Read the model definition and answer for the solid it produces. Units are mm, in the model's axes. A direction names the side the tool comes from. Round coordinates to 2 decimals unless told otherwise and drop trailing zeros. Order: outer loops, then holes, each group sorted by start corner. A loop starts at its lowest first (then second) coordinate and runs counter-clockwise, first axis right, second up.
from build123d import *

# Parameters (mm, degrees)
CYLINDER002_R     = 1.8
CYLINDER002_DEPTH = 10
ARRAY003_X_COUNT  = 2
ARRAY003_X_PITCH  = 75
ARRAY003_Y_COUNT  = 2
ARRAY003_Y_PITCH  = 31
BOX008_W          = 80.4
BOX008_H          = 36.4
BOX008_DEPTH      = 4.7
BOX_W             = 71.2
BOX_H             = 25
BOX_DEPTH         = 3.8


with BuildPart() as hole_clone:
    # Cylinder002 → Cylinder002 (new body)
    with BuildSketch(Plane(origin=(3.7, 3.7, 0), x_dir=(1, 0, 0), z_dir=(0, 0, 1))):
        Circle(CYLINDER002_R)
    extrude(amount=CYLINDER002_DEPTH)

    # Array003 X: hole clone ×2


with BuildPart() as hole_clone_1:
    add(hole_clone.part)
    with Locations(*[(i * ARRAY003_X_PITCH, 0, 0) for i in range(1, ARRAY003_X_COUNT)]):
        add(hole_clone.part)

    # Array003 Y: hole clone ×2


with BuildPart() as hole_clone_2:
    add(hole_clone_1.part)
    with Locations(*[(0, i * ARRAY003_Y_PITCH, 0) for i in range(1, ARRAY003_Y_COUNT)]):
        add(hole_clone_1.part)


with BuildPart() as hole_clone_3:
    # Body placement: moved
    add(hole_clone_2.part.moved(Location((-1, -1, 0))))


with BuildPart() as under_display:
    # Box008 → Box008 (new body)
    with BuildSketch(Plane.XY):
        with Locations((40.2, 18.2)):
            Rectangle(BOX008_W, BOX008_H)
    extrude(amount=BOX008_DEPTH)


with BuildPart() as f_16x2_lcd_mockup_clone:
    # Box → Box (new body)
    with BuildSketch(Plane(origin=(4.4, 5.2, 4.7), x_dir=(1, 0, 0), z_dir=(0, 0, 1))):
        with Locations((35.6, 12.5)):
            Rectangle(BOX_W, BOX_H)
    extrude(amount=BOX_DEPTH)

    # Fusion004: union under display
    add(under_display.part)

    # Cut: cut hole clone
    add(hole_clone_3.part, mode=Mode.SUBTRACT)


with BuildPart() as f_16x2_lcd_mockup_clone_1:
    # Body002 placement: moved
    add(f_16x2_lcd_mockup_clone.part.moved(Location((0, 22, 46))))


solid = f_16x2_lcd_mockup_clone_1.part
Q1. For faces 5 (the face through (75.6, 40, 53)), 6 (the face through (40, 52.2, 53)), 7 (the face through (4.4, 40, 53)), 8 (the face through (40, 27.2, 53)), 9 (the face through (40, 58.4, 48)), determine the directions among +Z, -Z, +X, -X, +Y, -Y from which every point of the face is accessible in a straight line to the end or side of a thin tool.
Outcome:
face 5: +Z, +X, +Y, -Y
face 6: +Z, +X, -X, +Y
face 7: +Z, -X, +Y, -Y
face 8: +Z, +X, -X, -Y
face 9: +Z, -Z, +X, -X, +Y
Q2. For a pull along Y with two mould halves and no side action, classify faces 1 (the face through (2.466, 26.485, 48.317)), 2 (the face through (40, 40, 54.5)), 3 (the face through (40, 22, 48)), 4 (the face through (76.272, 54.605, 48.317)) as released by +Y, released by -Y, zero draft, split by the parting line, or undercut.
Outcome:
face 1: undercut
face 2: zero draft
face 3: released by -Y
face 4: undercut
Q3. A cutting plane is placed at C-C, the plane y = 50.5. Give the vertices of the cut face in (x, z).
Outcome:
outline: (0, 46) - (80.4, 46) - (80.4, 50.7) - (75.6, 50.7) - (75.6, 54.5) - (4.4, 54.5) - (4.4, 50.7) - (0, 50.7) - close
Q4. Straight lines are drawn through the part: probe 1 along X at (y, z) = (24.7, 49.7); probe 2 along Y at (x, z) = (2.7, 48.65); probe 3 along Y at (x, z) = (35, 51.25). For each, find the intervals that lie inside material, in ascending order.
Outcome:
probe 1: x = 0 to 0.9, 4.5 to 75.9, 79.5 to 80.4
probe 2: y = 22 to 22.9, 26.5 to 53.9, 57.5 to 58.4
probe 3: y = 27.2 to 52.2
Q5. A cutting plane is placed at D-D, the plane z = 52.25. Give the vertices of the cut face in (x, y).
Outcome:
outline: (4.4, 27.2) - (75.6, 27.2) - (75.6, 52.2) - (4.4, 52.2) - close
Q6. A cutting plane is placed at A-A, the plane y = 55.7. Give the vertices of the cut face in (x, z).
Outcome:
outline: (0, 46) - (0.9, 46) - (0.9, 50.7) - (0, 50.7) - close; (4.5, 46) - (75.9, 46) - (75.9, 50.7) - (4.5, 50.7) - close; (79.5, 46) - (80.4, 46) - (80.4, 50.7) - (79.5, 50.7) - close
Q7. Flat-ended cylindrical pins translate along their axes: pin 1 (1.9 mm diameter, centred on y = 36.5, z = 52, fed in from -X); pin 2 (3 mm diameter, centred on x = 27, z = 53, fed in from -Y); pin 3 (6 mm diameter, centred on x = 2.7, y = 55.7, fed in from +Z). Find the tip coordinate at first contact, or state that the pin passes through.
Outcome:
pin 1: stops at x = 4.4
pin 2: stops at y = 27.2
pin 3: stops at z = 50.7
Q8. A cutting plane is placed at B-B, the plane x = 2.7. Give the vertices of the cut face in (y, z), plus the area to 3 significant figures.
Outcome:
outline: (22, 46) - (22.9, 46) - (22.9, 50.7) - (22, 50.7) - close; (26.5, 46) - (53.9, 46) - (53.9, 50.7) - (26.5, 50.7) - close; (57.5, 46) - (58.4, 46) - (58.4, 50.7) - (57.5, 50.7) - close
area: 137 mm2
